Can you work these out from the model? Positions are in its coordinate system, mm. Coordinates: 2 decimals unless noted, no trailing zeros. Loops run counter-clockwise (first coordinate to the right, second up) from the corner with the lowest first, then second, coordinate; pieces in that order, holes last. Notation, with made-up numbers: (54, -28.5) -> (106, -28.5) arc R28 cw to (106, -4.5) -> close; hole circle Ø7 at (-1.5, 77). An arc over 180 degrees is marked (long way). Use one line per item in the form item = value. Start each with the question number.
(1) I need wall thicknesses on line 1 (Z direction, x = 2.15, y = 0); line 2 (Y direction, x = 1.8, z = -5); line 3 (Y direction, x = 1.8, z = 7). Which ranges of each line are inside material? Lowest first, please. Write a range as [from, to].
(2) Imagine slicing it at D-D (y = 5.5). List the corners of the cut face in (x, z) for me.
(3) Imagine slicing it at A-A (z = 0). List the corners of the cut face in (x, y) for me.
(4) Imagine slicing it at B-B (y = 75). List the corners of the cut face in (x, z) for me, plus the area to 3 significant figures.
(5) Thinking about a two-plate mould opening in Z: for faces 1 (the cylindrical face through (2.504, -14.274, 0.628)), 2 (the flat face through (3, 43, -25.4)), 3 (the flat face through (3, 44, 25.4)), 4 (the cylindrical face through (2.504, 67.217, 0.628)), which applies, released by +Z, released by -Z, zero draft, split by the parting line, or undercut?
(6) Imagine slicing it at C-C (x = 3.25). List the corners of the cut face in (y, z) for me (1 decimal), plus the area to 3 significant figures.
```python
from build123d import *

# Parameters (mm, degrees)
F0_R     = 14.2875
F1_DEPTH = 5.08


with BuildPart() as f1:
    # F0 (on Right) → F1 (new body)
    with BuildSketch(Plane.YZ):
        with BuildLine():
            Line((86.49098, 25.4), (0, 25.4))
            ThreePointArc((0, 25.4), (-25.4, 0), (0, -25.4))
            Line((0, -25.4), (86.49098, -25.4))
            ThreePointArc((86.49098, -25.4), (100.633116, -19.542136), (106.49098, -5.4))
            Line((106.49098, -5.4), (106.49098, 5.4))
            ThreePointArc((106.49098, 5.4), (100.633116, 19.542136), (86.49098, 25.4))
        make_face()
        Circle(F0_R, mode=Mode.SUBTRACT)
        with Locations((81.49098, 0)):
            Circle(F0_R, mode=Mode.SUBTRACT)
    extrude(amount=F1_DEPTH)


solid = f1.part
```
Worked out:
q1.line_1 = [-25.4, -14.29], [14.29, 25.4]
q1.line_2 = [-24.9, -13.38], [13.38, 68.11], [94.88, 106.49]
q1.line_3 = [-24.42, -12.46], [12.46, 69.04], [93.95, 106.43]
q2.outline = (0, -25.4) -> (5.08, -25.4) -> (5.08, -13.19) -> (0, -13.19) -> close; (0, 13.19) -> (5.08, 13.19) -> (5.08, 25.4) -> (0, 25.4) -> close
q3.outline = (0, -25.4) -> (5.08, -25.4) -> (5.08, -14.29) -> (0, -14.29) -> close; (0, 14.29) -> (5.08, 14.29) -> (5.08, 67.2) -> (0, 67.2) -> close; (0, 95.78) -> (5.08, 95.78) -> (5.08, 106.49) -> (0, 106.49) -> close
q4.outline = (0, -25.4) -> (5.08, -25.4) -> (5.08, -12.73) -> (0, -12.73) -> close; (0, 12.73) -> (5.08, 12.73) -> (5.08, 25.4) -> (0, 25.4) -> close
q4.area = 129 mm2
q5.face_1 = undercut
q5.face_2 = released by -Z
q5.face_3 = released by +Z
q5.face_4 = undercut
q6.outline = (0, -25.4) -> (86.5, -25.4) arc R20 ccw to (106.5, -5.4) -> (106.5, 5.4) arc R20 ccw to (86.5, 25.4) -> (0, 25.4) arc R25.4 ccw to start; hole circle Ø28.6 at (0, 0); hole circle Ø28.6 at (81.5, 0)
q6.area = 4,970 mm2
